The listing builds one solid part. Answer for the finished solid, in the listing's coordinates (mm). Face numbers are marked on the shaded views. Round coordinates to 2 decimals unless told otherwise and drop trailing zeros. Loops run counter-clockwise (first coordinate to the right, second up) from the corner with the lowest first, then second, coordinate; pieces in that order, holes last. Notation, with made-up numbers: (1.5, 27.25) -> (53.5, 27.25) arc R20 ccw to (53.5, 61.25) -> close; hole circle Ø6 at (-7, 49.25). An arc over 180 degrees is marked (long way). Use a Markdown table: item, result. Add a question column.
Q1. Given pin 1 Ø2 at (y, z) = (-1.5, -58) entering from -X; pin 2 Ø2 at (y, z) = (-2, -41.5) entering from +X; pin 3 Ø1.5 at (x, y) = (68.5, -2) entering from +Z, each flat-ended and moving along its own axis, determine where each tip first touches the part or whether it passes through.
Q2. Section A-A on x = 100 is taken. Give the vertices of the cut face in (y, z), then the cut area to 3 significant figures.
Q3. Section D-D on y = -1.25 is taken. Give the vertices of the cut face in (x, z).
Q4. For a pull along X with two mould halves and no side action, classify the marked faces 1 and 2 as released by +X, released by -X, zero draft, split by the parting line, or undercut.
Q5. Consider line 1 (X direction, y = 0.15, z = -36); line 2 (X direction, y = 0.2, z = -87); line 3 (X direction, y = -2, z = -90.5). Determine where each line is inside the solid, lowest interval first.
Q6. Section B-B on z = -33 is taken. Give the vertices of the cut face in (x, y), then the cut area to 3 significant figures.
Q7. Section C-C on x = 44 is taken. Give the vertices of the cut face in (y, z).
Autodesk Inventor part; units mm, degrees
ref_plane "YZ Plane" through (0, 0, 0) normal (1, 0, 0) x (0, 1, 0)
ref_plane "XZ Plane" through (0, 0, 0) normal (0, 1, 0) x (-1, 0, 0)
ref_plane "XY Plane" through (0, 0, 0) normal (0, 0, 1) x (1, 0, 0)
sketch "Sketch1" plane through (0, 0, 0) normal (0, 1, 0) x (-1, 0, 0)
  circle A0 centre (-103.3712, -13.8328) radius 2.5
  circle A1 centre (-103.3712, -93.8328) radius 2.5
  circle A2 centre (-78.3712, -13.8328) radius 2.5
  circle A3 centre (-78.3712, -93.8328) radius 2.5
  line L0 (-8.8712, -9.8328) -> (-107.3712, -9.8328)
  line L1 (-107.3712, -9.8328) -> (-107.3712, -98.8828)
  line L2 (-107.3712, -98.8828) -> (-8.8712, -98.8828)
  line L3 (-8.8712, -98.8828) -> (-8.8712, -69.8328)
  line L4 (-5.8712, -69.8328) -> (-8.8712, -69.8328)
  line L5 (-5.8712, -57.8328) -> (-5.8712, -69.8328)
  line L6 (-5.8712, -57.8328) -> (-8.8712, -57.8328)
  line L7 (-8.8712, -57.8328) -> (-8.8712, -9.8328)
  line L8 (-8.8712, -57.8328) -> (-6.8712, -57.8328)
  line L9 (-6.8712, -57.8328) -> (-6.8712, -69.8328)
  line L10 (-6.8712, -69.8328) -> (-8.8712, -69.8328)
  line L11 (-8.8712, -69.8328) -> (-8.8712, -98.8828)
  line L12 (-8.8712, -98.8828) -> (-107.3712, -98.8828)
  line L13 (-107.3712, -98.8828) -> (-107.3712, -9.8328)
  line L14 (-107.3712, -9.8328) -> (-8.8712, -9.8328)
  line L15 (-8.8712, -9.8328) -> (-8.8712, -57.8328)
  line L16 (-5.8712, -6.8328) -> (-110.3712, -6.8328)
  line L17 (-110.3712, -6.8328) -> (-110.3712, -101.8828)
  line L18 (-110.3712, -101.8828) -> (-5.8712, -101.8828)
  line L19 (-5.8712, -101.8828) -> (-5.8712, -6.8328)
  line L20 (-103.3712, -93.8328) -> (-78.3712, -93.8328) construction
  line L21 (-78.3712, -93.8328) -> (-78.3712, -13.8328) construction
  line L22 (-78.3712, -13.8328) -> (-103.3712, -13.8328) construction
  line L23 (-103.3712, -13.8328) -> (-103.3712, -93.8328) construction
  line L24 (-90.8712, -93.8328) -> (-90.8712, -13.8328) construction
  line L25 (-103.3712, -53.8328) -> (-78.3712, -53.8328) construction
  line L26 (-76.8712, -89.8328) -> (-104.8712, -89.8328)
  line L27 (-104.8712, -89.8328) -> (-104.8712, -17.8328)
  line L28 (-104.8712, -17.8328) -> (-76.8712, -17.8328)
  line L29 (-76.8712, -17.8328) -> (-76.8712, -89.8328)
  line L30 (-76.8712, -89.8328) -> (-104.8712, -17.8328) construction
  line L31 (-104.8712, -89.8328) -> (-76.8712, -17.8328) construction
  line L32 (-9.0712, -58.0328) -> (-7.0712, -58.0328)
  line L33 (-7.0712, -58.0328) -> (-7.0712, -69.6328)
  line L34 (-7.0712, -69.6328) -> (-9.0712, -69.6328)
  line L35 (-9.0712, -69.6328) -> (-9.0712, -98.6828)
  line L36 (-9.0712, -98.6828) -> (-107.1712, -98.6828)
  line L37 (-107.1712, -98.6828) -> (-107.1712, -10.0328)
  line L38 (-107.1712, -10.0328) -> (-9.0712, -10.0328)
  line L39 (-9.0712, -10.0328) -> (-9.0712, -58.0328)
  line L40 (-10.5712, -59.5328) -> (-8.5712, -59.5328)
  line L41 (-8.5712, -59.5328) -> (-8.5712, -68.1328)
  line L42 (-8.5712, -68.1328) -> (-10.5712, -68.1328)
  line L43 (-10.5712, -68.1328) -> (-10.5712, -97.1828)
  line L44 (-10.5712, -97.1828) -> (-105.6712, -97.1828)
  line L45 (-105.6712, -97.1828) -> (-105.6712, -11.5328)
  line L46 (-105.6712, -11.5328) -> (-10.5712, -11.5328)
  line L47 (-10.5712, -11.5328) -> (-10.5712, -59.5328)
  line L48 (-10.5712, -11.5328) -> (-76.1712, -11.5328)
  line L49 (-76.1712, -11.5328) -> (-76.1712, -77.1328)
  line L50 (-76.1712, -77.1328) -> (-10.5712, -77.1328)
  line L51 (-10.5712, -77.1328) -> (-10.5712, -11.5328)
  line L52 (-11.5712, -76.1328) -> (-75.1712, -76.1328)
  line L53 (-75.1712, -76.1328) -> (-75.1712, -12.5328)
  line L54 (-75.1712, -12.5328) -> (-11.5712, -12.5328)
  line L55 (-11.5712, -12.5328) -> (-11.5712, -76.1328)
  line L56 (-76.1712, -77.1328) -> (-10.5712, -77.1328)
  line L57 (-10.5712, -77.1328) -> (-10.5712, -97.1828)
  line L58 (-10.5712, -97.1828) -> (-76.1712, -97.1828)
  line L59 (-76.1712, -97.1828) -> (-76.1712, -77.1328)
  line L60 (-43.3712, -97.1828) -> (-43.3712, -77.1328) construction
  line L61 (-10.5712, -87.1578) -> (-76.1712, -87.1578) construction
  line L62 (-40.1712, -90.3578) -> (-46.5712, -90.3578)
  line L63 (-46.5712, -90.3578) -> (-46.5712, -83.9578)
  line L64 (-46.5712, -83.9578) -> (-40.1712, -83.9578)
  line L65 (-40.1712, -83.9578) -> (-40.1712, -90.3578)
  line L66 (-40.1712, -90.3578) -> (-46.5712, -83.9578) construction
  line L67 (-46.5712, -90.3578) -> (-40.1712, -83.9578) construction
  line L68 (-41.1212, -89.4078) -> (-45.6212, -89.4078)
  line L69 (-45.6212, -89.4078) -> (-45.6212, -84.9078)
  line L70 (-45.6212, -84.9078) -> (-41.1212, -84.9078)
  line L71 (-41.1212, -84.9078) -> (-41.1212, -89.4078)
  line L72 (-41.1212, -89.4078) -> (-45.6212, -84.9078) construction
  line L73 (-45.6212, -89.4078) -> (-41.1212, -84.9078) construction
  point P0 (0, 0)
  point P1 (-90.8712, -53.8328)
  point P2 (-105.6712, -94.8126)
  point P3 (-105.6712, -92.853)
  point P4 (-105.6712, -14.8126)
  point P5 (-105.6712, -12.853)
  point P6 (-104.351, -11.5328)
  point P7 (-102.3914, -11.5328)
  point P8 (-79.351, -11.5328)
  point P9 (-77.3914, -11.5328)
  point P10 (-43.3712, -87.1578)
  dimension "d0" = 28
  dimension "d1" = 72
  dimension "d2" = 0.2
  dimension "d3" = 1.5
  dimension "d10" = 65.6
  dimension "d11" = 65.6
  dimension "d12" = 1
  dimension "d15" = 6.4
  dimension "d16" = 6.4
  dimension "d17" = 4.5
  dimension "d18" = 4.5
extrude "Extrusion1" add sketch "Sketch1" against normal blind 3 contours L46 A0 | A0 L45 | A2 L46 | L45 A1 | L32 L33 L34 L35 L36 L37 L38 L39 picked at (-105.721, -93.6661)
extrude "Extrusion2" add sketch "Sketch1" along normal blind 2 contours A0 L45 L46 | A0 L46 A2 L49 L59 A3 L44 L45 A1 | L46 A0 | A0 L45 | A0 L45 L46 | L46 A2 L49 | A2 L46 | L45 A1 | A1 L45 | L46 L49 A2 | L49 A2 | A2 L49 L46 L47 L51 L43 L50 | L50 L43 L44 L59 A3 | L59 A3 | A3 L59 | L40 L41 L42 L51 | L7 L6 L9 L4 L3 L2 L1 L0 | L0 L1 L2 L3 L4 L19 L18 L17 L16 L6 L7 | L6 L5 L4 L9 | L26 L27 L28 L29 | L32 L33 L34 L35 L36 L37 L38 L39 | L52 L53 L54 L55 | L62 L63 L64 L65 | L68 L69 L70 L71
extrude "Extrusion3" cut sketch "Sketch1" along normal up to surface (2 mm away) contours L26 L27 L28 L29
extrude "Extrusion4" cut sketch "Sketch1" along normal up to surface (2 mm away) contours L52 L53 L54 L55
extrude "Extrusion5" cut sketch "Sketch1" along normal up to surface (2 mm away) contours L68 L69 L70 L71
extrude "Extrusion6" cut sketch "Sketch1" along normal blind 1 contours L62 L63 L64 L65
fillet "Fillet1" radius 3.175 4 edges at (5.8712, 1, -101.8828) (5.8712, 1, -6.8328) (110.3712, 1, -6.8328) (110.3712, 1, -101.8828)
properties part number "EnclosureLid"
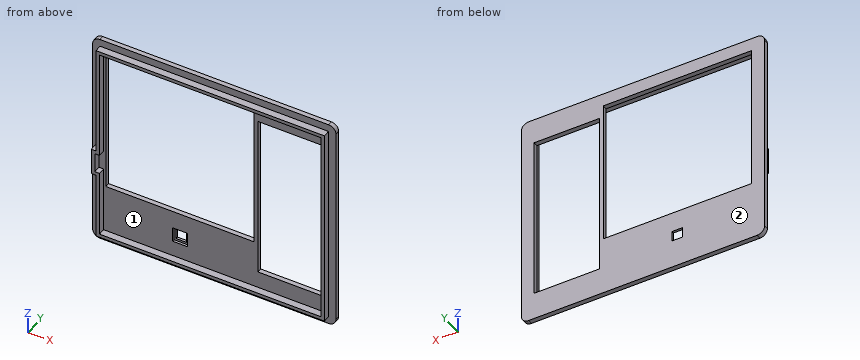
Checked values:
| question | item | result |
|---|---|---|
| 1 | pin 1 | stops at x = 7.07 |
| 1 | pin 2 | stops at x = 107.17 |
| 1 | pin 3 | stops at z = -10.03 |
| 2 | outline | (-3, -98.68) -> (0, -98.68) -> (0, -101.88) -> (2, -101.88) -> (2, -89.83) -> (0, -89.83) -> (0, -97.18) -> (-3, -97.18) -> close; (-3, -11.53) -> (0, -11.53) -> (0, -17.83) -> (2, -17.83) -> (2, -6.83) -> (0, -6.83) -> (0, -10.03) -> (-3, -10.03) -> close |
| 2 | area | 55.1 mm2 |
| 3 | outline | (7.07, -69.63) -> (9.07, -69.63) -> (9.07, -98.68) -> (107.17, -98.68) -> (107.17, -10.03) -> (9.07, -10.03) -> (9.07, -58.03) -> (7.07, -58.03) -> close; hole (8.57, -68.13) -> (10.57, -68.13) -> (10.57, -97.18) -> (105.67, -97.18) -> (105.67, -11.53) -> (10.57, -11.53) -> (10.57, -59.53) -> (8.57, -59.53) -> close |
| 4 | face 1 | undercut |
| 4 | face 2 | zero draft |
| 5 | line 1 | x = 5.87 to 11.57, 75.17 to 76.87, 104.87 to 110.37 |
| 5 | line 2 | x = 5.87 to 40.17, 46.57 to 76.87, 104.87 to 110.37 |
| 5 | line 3 | x = 9.07 to 10.57, 105.67 to 107.17 |
| 6 | outline | (5.87, 0) -> (9.07, 0) -> (9.07, -3) -> (10.57, -3) -> (10.57, 0) -> (11.57, 0) -> (11.57, 2) -> (5.87, 2) -> close; (75.17, 0) -> (76.87, 0) -> (76.87, 2) -> (75.17, 2) -> close; (104.87, 0) -> (105.67, 0) -> (105.67, -3) -> (107.17, -3) -> (107.17, 0) -> (110.37, 0) -> (110.37, 2) -> (104.87, 2) -> close |
| 6 | area | 34.8 mm2 |
| 7 | outline | (-3, -98.68) -> (0, -98.68) -> (0, -101.88) -> (2, -101.88) -> (2, -89.41) -> (1, -89.41) -> (1, -90.36) -> (0, -90.36) -> (0, -97.18) -> (-3, -97.18) -> close; (-3, -11.53) -> (0, -11.53) -> (0, -12.53) -> (2, -12.53) -> (2, -6.83) -> (0, -6.83) -> (0, -10.03) -> (-3, -10.03) -> close; (0, -83.96) -> (1, -83.96) -> (1, -84.91) -> (2, -84.91) -> (2, -76.13) -> (0, -76.13) -> close |
